Read the model definition and answer for the solid it produces. Units are mm, in the model's axes. A direction names the side the tool comes from. Give positions to 0.01 mm unless a question says otherwise; leave off trailing zeros. Order: outer loops, then holes, each group sorted by start corner. A loop starts at its lowest first (then second) coordinate and runs counter-clockwise, first axis right, second up. Notation, with made-up numbers: (10, 16) - (15, 16) arc R22 cw to (15, 48) - close; hole circle Ø2 at (50.5, -3.75). An arc over 180 degrees is marked (long way). Use a Markdown table: item, result. Add a question column.
1. Which of the six approach directions +Z, -Z, +X, -X, +Y, -Y give full straight-line access (tool end or side, diameter ignored) to faces 4 (the flat face through (0, 12, -10)), 5 (the flat face through (0, 20, -3)), 6 (the cylindrical face through (0.06, 14.626, -10.07)), 7 (the cylindrical face through (0.06, 56.374, 13.07)), 8 (the cylindrical face through (-1.34, 8.93, 0.3))?
2. A cutting plane is placed at D-D on z = 0. Determine the outline of the cut face in (x, y) (3 decimals).
3. Flat-ended cylindrical pins translate along their axes: P1, Ø1.6, axis at x = 0, y = 55, coming from the -Z side; P2, Ø0.8, axis at x = 0.5, z = 0.5, coming from the -Y side; P3, Ø2, axis at x = 0, y = 54.5, coming from the -Z side; P4, Ø3, axis at x = -3.5, z = -5.5, coming from the +Y side. Find the tip coordinate at first contact, or state that the pin passes through.
4. A cutting plane is placed at A-A on z = -8.5. Determine the outline of the cut face in (x, y) (3 decimals).
5. Consider L1, parallel to X at y = 9, z = 0 (3 decimals); L2, parallel to Z at x = 6, y = 35; L3, parallel to Y at x = 5.75, z = 10.5. Determine where each line is inside the solid, lowest interval first.
6. For a pull along Z with two mould halves and no side action, classify faces 1 (the cylindrical face through (-0.14, 49.289, 13.196)), 2 (the flat face through (0, 14, 0)), 3 (the cylindrical face through (0, 59, 2)) as released by +Z, released by -Z, zero draft, split by the parting line, or undercut.
7. A cutting plane is placed at B-B on y = 16. Determine the outline of the cut face in (x, z) (3 decimals).
```python
from build123d import *

# Parameters (mm, degrees)
PAD_DEPTH       = 10
SKETCH001_R     = 1.375
POCKET_DEPTH    = 10
PAD001_DEPTH    = 33
SKETCH003_R     = 1.375
POCKET001_DEPTH = 10
SKETCH004_R     = 1.375
POCKET002_DEPTH = 10
FILLET_1_R      = 9
FILLET_2_R      = 6
CHAMFER_SIZE    = 5


with BuildPart() as part:
    # Sketch → Pad (new body, symmetric)
    with BuildSketch(Plane.YZ):
        Polygon((4, 4), (17, 4), (17, 18), (54, 18), (54, -15), (51, -15), (51, 15), (20, 15), (20, -15), (12, -15), (12, -4), (4, -4), align=None)
    extrude(amount=PAD_DEPTH, both=True)

    # Sketch001 → Pocket (cut)
    with BuildSketch(Plane(origin=(0, 4, 0), x_dir=(0, 0, -1), z_dir=(0, -1, 0))):
        Circle(SKETCH001_R)
    extrude(amount=-POCKET_DEPTH, mode=Mode.SUBTRACT)

    # Sketch002 → Pad001 (new body)
    with BuildSketch(Plane(origin=(0, 0, 18), x_dir=(0, -1, 0), z_dir=(0, 0, 1))):
        with BuildLine():
            ThreePointArc((-58.492889, 1.949289), (-59, 0), (-58.492889, -1.949289))
            Line((-54, -10), (-58.492889, -1.949289))
            Line((-54, 10), (-54, -10))
            Line((-58.492889, 1.949289), (-54, 10))
        make_face()
    extrude(amount=-PAD001_DEPTH)

    # Sketch003 → Pocket001 (cut)
    with BuildSketch(Plane(origin=(0, 0, 18), x_dir=(0, -1, 0), z_dir=(0, 0, 1))):
        with Locations((-55, 0)):
            Circle(SKETCH003_R)
    extrude(amount=-POCKET001_DEPTH, mode=Mode.SUBTRACT)

    # Sketch004 → Pocket002 (cut)
    with BuildSketch(Plane.YX.offset(15)):
        with Locations((55, 0)):
            Circle(SKETCH004_R)
        with Locations((16, 0)):
            Circle(SKETCH004_R)
    extrude(amount=-POCKET002_DEPTH, mode=Mode.SUBTRACT)

    # Fillet 1
    fillet_1_edges = [part.edges().sort_by_distance(p)[0] for p in [
        (0, 17, 18),
    ]]
    fillet(fillet_1_edges, radius=FILLET_1_R)

    # Fillet 2
    fillet_2_edges = [part.edges().sort_by_distance(p)[0] for p in [
        (0, 20, 15),
        (0, 51, 15),
    ]]
    fillet(fillet_2_edges, radius=FILLET_2_R)

    # Chamfer
    chamfer_edges = [part.edges().sort_by_distance(p)[0] for p in [
        (-10, 52.5, -15),
        (-10, 16, -15),
        (10, 52.5, -15),
        (10, 16, -15),
    ]]
    chamfer(chamfer_edges, length=CHAMFER_SIZE)


solid = part.part
```
Output values:
| question | item | result |
|---|---|---|
| 1 | face 4 | -Z, +X, -X, -Y |
| 1 | face 5 | -Z, +X, -X |
| 1 | face 6 | -Z |
| 1 | face 7 | +Z |
| 1 | face 8 | -Y |
| 2 | outline | (-10, 4) - (-1.375, 4) - (-1.375, 14) - (1.375, 14) - (1.375, 4) - (10, 4) - (10, 20) - (-10, 20) - close; (-10, 51) - (10, 51) - (10, 54) - (1.949, 58.493) arc R4 ccw to (-1.949, 58.493) - (-10, 54) - close |
| 3 | P1 | z = -5 |
| 3 | P2 | y = 14 |
| 3 | P3 | z = -15 |
| 3 | P4 | y = 58.46 |
| 4 | outline | (-10, 12) - (10, 12) - (10, 20) - (-10, 20) - close; (-10, 51) - (10, 51) - (10, 54) - (1.949, 58.493) arc R4 ccw to (-1.949, 58.493) - (-10, 54) - close; hole circle Ø2.75 at (0, 16); hole circle Ø2.75 at (0, 55) |
| 5 | L1 | -10 to -1.375, 1.375 to 10 |
| 5 | L2 | 15 to 18 |
| 5 | L3 | 17.13 to 20.19, 50.81 to 56.37 |
| 6 | face 1 | released by -Z |
| 6 | face 2 | undercut |
| 6 | face 3 | zero draft |
| 7 | outline | (-10, -10) - (-5, -15) - (-1.375, -15) - (-1.375, -5) - (1.375, -5) - (1.375, -15) - (5, -15) - (10, -10) - (10, 4) - (-10, 4) - close |
